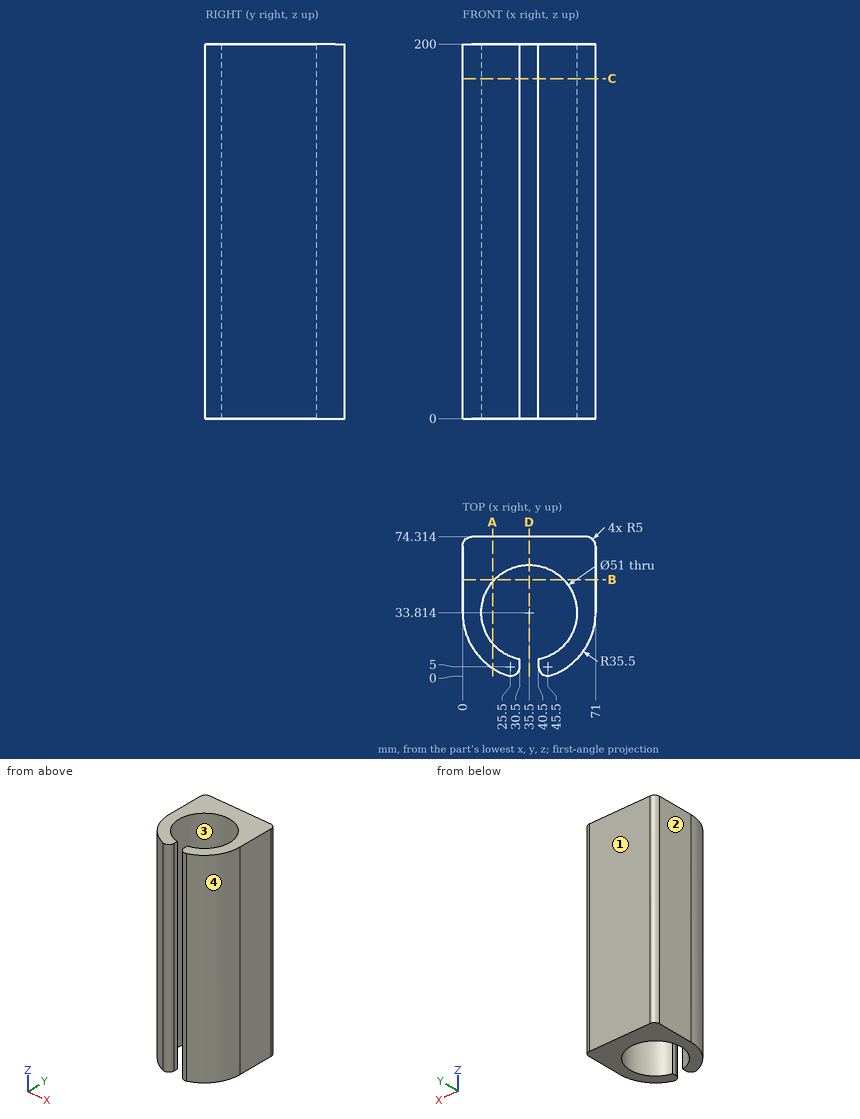
Geometry: see drawing. Coordinates: mm, zero at the bounding-box minimum. Round coordinates to 2 decimals unless told otherwise and drop trailing zeros. Order: outer loops, then holes, each group sorted by start corner. A loop starts at its lowest first (then second) coordinate and runs counter-clockwise, first axis right, second up. Notation, with made-up numbers: (80.25, 67) - (85.25, 67) arc R15 ccw to (85.25, 85) - close; hole circle Ø4 at (-1, -17.5). An arc over 180 degrees is marked (long way). Use a Markdown table: item, result. Add a question column.
1. Section query B-B (y = 51.5). Return the cut outline in (x, z).
2. Line query: probe 1 along Y at (x, z) = (35.5, 88.5); probe 2 along X at (y, z) = (45, 138); probe 3 along Y at (x, z) = (19.5, 161.5). Output: solid intervals per line, ascending.
3. Mould query, pull axis X, two halves, no side actions, for the marked faces 1, 2, 3 and 4. Classes: +X half, -X half, draft (parallel to the pull), parting line (faces both ways), or undercut.
4. First-contact query: pin 1 (2 mm diameter, centred on x = 56.5, z = 105.5, fed in from -Y); pin 2 (4 mm diameter, centred on x = 40.5, z = 168, fed in from -Y); pin 3 (5 mm diameter, centred on y = 21, z = 142.5, fed in from +X). Flat tips, straight axial feed; report the tip coordinate or a pass-through.
5. Section query D-D (x = 35.5). Return the cut outline in (y, z), then the cut area to 3 significant figures.
6. Section query A-A (x = 16). Return the cut outline in (y, z), then the cut area to 3 significant figures.
7. Section query C-C (z = 181.5). Return the cut outline in (x, y), then the cut area to 3 significant figures.
Derived:
| question | item | result |
|---|---|---|
| 1 | outline | (0, 0) - (17.13, 0) - (17.13, 200) - (0, 200) - close; (53.87, 0) - (71, 0) - (71, 200) - (53.87, 200) - close |
| 2 | probe 1 | 59.31 to 74.31 |
| 2 | probe 2 | 0 to 12.58, 58.42 to 71 |
| 2 | probe 3 | 2.12 to 13.96, 53.67 to 74.31 |
| 3 | face 1 | draft |
| 3 | face 2 | -X half |
| 3 | face 3 | undercut |
| 3 | face 4 | +X half |
| 4 | pin 1 | y = 4.48 |
| 4 | pin 2 | y = 1 |
| 4 | pin 3 | x = 69.47 |
| 5 | outline | (59.31, 0) - (74.31, 0) - (74.31, 200) - (59.31, 200) - close |
| 5 | area | 3,000 mm2 |
| 6 | outline | (4.15, 0) - (17.38, 0) - (17.38, 200) - (4.15, 200) - close; (50.25, 0) - (74.31, 0) - (74.31, 200) - (50.25, 200) - close |
| 6 | area | 7,460 mm2 |
| 7 | outline | (0, 33.81) arc R35.5 ccw to (23.86, 0.28) arc R5 ccw to (30.5, 5) - (30.5, 8.81) arc R25.5 cw (long way) to (40.5, 8.81) - (40.5, 5) arc R5 ccw to (47.14, 0.28) arc R35.5 ccw to (71, 33.81) - (71, 69.31) arc R5 ccw to (66, 74.31) - (5, 74.31) arc R5 ccw to (0, 69.31) - close |
| 7 | area | 2,680 mm2 |
